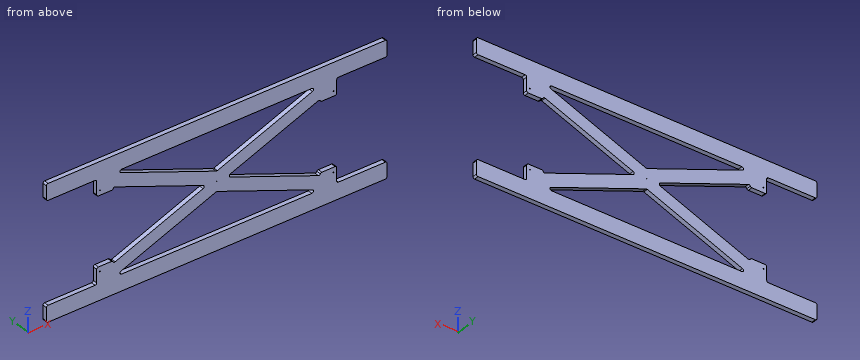
```python
from build123d import *

# Parameters (mm, degrees)
SKETCH1_W                    = 1333.5
SKETCH1_H                    = 520.7
BOSS_EXTRUDE1_DEPTH          = 17.78
FILLET1_R                    = 6.35
F_1_8_0_125_DIAMETER_HOLE1_D = 3.175
SKETCH5_W                    = 152.4
SKETCH5_H                    = 393.7
CUT_EXTRUDE1_DEPTH           = 18.78
FILLET2_R                    = 6.35
SKETCH6_W                    = 50.8
SKETCH6_H                    = 393.7
SKETCH6_W_2                  = 63.5
SKETCH6_H_2                  = 266.7
CUT_EXTRUDE2_DEPTH           = 18.78
FILLET3_R                    = 6.35


with BuildPart() as part:
    # Sketch1 → Boss-Extrude1 (new body)
    with BuildSketch(Plane(origin=(0, 0, 0), x_dir=(1, 0, 0), z_dir=(0, 1, 0))):
        Rectangle(SKETCH1_W, SKETCH1_H)
    extrude(amount=BOSS_EXTRUDE1_DEPTH)

    # Fillet1
    fillet1_edges = [part.edges().sort_by_distance(p)[0] for p in [
        (666.75, 8.89, 260.35),
        (-666.75, 8.89, 260.35),
        (-666.75, 8.89, -260.35),
        (666.75, 8.89, -260.35),
    ]]
    fillet(fillet1_edges, radius=FILLET1_R)

    # 1/8 (0.125) Diameter Hole1 (through all)
    with Locations(Plane(origin=(0, 17.78, 0), x_dir=(1, 0, 0), z_dir=(0, 1, 0))):
        with Locations((0, 0), (457.2, 152.4), (-457.2, -152.4), (-457.2, 152.4), (457.2, -152.4)):
            Hole(F_1_8_0_125_DIAMETER_HOLE1_D / 2)

    # Sketch5 → Cut-Extrude1 (cut, through all)
    with BuildSketch(Plane(origin=(0, 17.78, 0), x_dir=(1, 0, 0), z_dir=(0, 1, 0))):
        Polygon((-406.4, 196.85), (406.4, 196.85), (0, 38.1), align=None)
        Polygon((0, -38.1), (-406.4, -196.85), (406.4, -196.85), align=None)
        Polygon((406.4, 143.8671875), (406.4, -143.8671875), (38.1, 0), align=None)
        Polygon((-406.4, 143.8671875), (-38.1, 0), (-406.4, -143.8671875), align=None)
        with Locations((546.1, 0)):
            Rectangle(SKETCH5_W, SKETCH5_H)
        with Locations((-546.1, 0)):
            Rectangle(SKETCH5_W, SKETCH5_H)
    extrude(amount=-CUT_EXTRUDE1_DEPTH, mode=Mode.SUBTRACT)

    # Fillet2
    fillet2_edges = [part.edges().sort_by_distance(p)[0] for p in [
        (-406.4, 8.89, 143.8671875),
        (-406.4, 8.89, -143.8671875),
        (-38.1, 8.89, 0),
        (622.3, 8.89, -196.85),
        (622.3, 8.89, 196.85),
        (469.9, 8.89, 196.85),
        (469.9, 8.89, -196.85),
        (0, 8.89, 38.1),
        (406.4, 8.89, 196.85),
        (-406.4, 8.89, 196.85),
        (38.1, 8.89, 0),
        (406.4, 8.89, -143.8671875),
        (406.4, 8.89, 143.8671875),
        (406.4, 8.89, -196.85),
        (0, 8.89, -38.1),
        (-406.4, 8.89, -196.85),
        (-469.9, 8.89, -196.85),
        (-469.9, 8.89, 196.85),
        (-622.3, 8.89, 196.85),
        (-622.3, 8.89, -196.85),
    ]]
    fillet(fillet2_edges, radius=FILLET2_R)

    # Sketch6 → Cut-Extrude2 (cut, through all)
    with BuildSketch(Plane(origin=(0, 17.78, 0), x_dir=(1, 0, 0), z_dir=(0, 1, 0))):
        with Locations((641.35, 0)):
            Rectangle(SKETCH6_W, SKETCH6_H)
        with Locations((-641.35, 0)):
            Rectangle(SKETCH6_W, SKETCH6_H)
        with Locations((-438.15, 0)):
            Rectangle(SKETCH6_W_2, SKETCH6_H_2)
        with Locations((438.15, 0)):
            Rectangle(SKETCH6_W_2, SKETCH6_H_2)
    extrude(amount=-CUT_EXTRUDE2_DEPTH, mode=Mode.SUBTRACT)

    # Fillet3
    fillet3_edges = [part.edges().sort_by_distance(p)[0] for p in [
        (-666.75, 8.89, 196.85),
        (-666.75, 8.89, -196.85),
        (666.75, 8.89, -196.85),
        (666.75, 8.89, 196.85),
        (-406.4, 8.89, 133.35),
        (-406.4, 8.89, -133.35),
        (-469.9, 8.89, 133.35),
        (-469.9, 8.89, -133.35),
        (469.9, 8.89, -133.35),
        (406.4, 8.89, -133.35),
        (469.9, 8.89, 133.35),
        (406.4, 8.89, 133.35),
    ]]
    fillet(fillet3_edges, radius=FILLET3_R)


solid = part.part
```
Input: part model. Units: mm. Frame: model coordinates. Coordinates: 2 decimals unless noted, no trailing zeros. Loops run counter-clockwise (first coordinate to the right, second up) from the corner with the lowest first, then second, coordinate; pieces in that order, holes last. Notation, with made-up numbers: (29, 9.5) -> (46, 9.5) arc R33 cw to (46, 42.5) -> close; hole circle Ø1 at (46, 30.25). An arc over 180 degrees is marked (long way). Use a Markdown table: item, result.
1) Cut plane C-C (y = 14.5). Give the number of separate pieces and of enclosed holes in the cut face, then the cut area to 3 significant figures.
Results found:
| item | result |
|---|---|
| separate pieces | 1 |
| enclosed holes | 7 |
| area | 271,000 mm2 |
2) Cut plane B-B (x = -297). Return the cut outline in (y, z), then the cut area to 3 significant figures.
Results found:
| item | result |
|---|---|
| outline | (0, -260.35) -> (17.78, -260.35) -> (17.78, -196.85) -> (0, -196.85) -> close; (0, -154.12) -> (17.78, -154.12) -> (17.78, -101.13) -> (0, -101.13) -> close; (0, 101.13) -> (17.78, 101.13) -> (17.78, 154.12) -> (0, 154.12) -> close; (0, 196.85) -> (17.78, 196.85) -> (17.78, 260.35) -> (0, 260.35) -> close |
| area | 4,140 mm2 |
3) Cut plane D-D (z = 172.5). Return the cut outline in (x, y).
Results found:
| item | result |
|---|---|
| outline | (-469.9, 0) -> (-344.06, 0) -> (-344.06, 17.78) -> (-469.9, 17.78) -> close; (344.06, 0) -> (469.9, 0) -> (469.9, 17.78) -> (344.06, 17.78) -> close |
4) Material intervals for line 1 along Z through (x, y) = (-457.2, 5.75); line 2 along Z through (x, y) = (130, 8); line 3 along Z through (x, y) = (9, 5.5), sorted ascending. Write a range as from..to.
Results found:
| item | result |
|---|---|
| line 1 | z = -260.35..-153.99, -150.81..-133.35, 133.35..150.81, 153.99..260.35 |
| line 2 | z = -260.35..-196.85, -88.88..-35.9, 35.9..88.88, 196.85..260.35 |
| line 3 | z = -260.35..-196.85, -41.62..41.62, 196.85..260.35 |
5) Contact query for flat-ended pins moving along their axis: pin 1 (2.5 mm diameter, centred on x = 457.2, z = -152.4, fed in from -Y); pin 2 (3 mm diameter, centred on y = 8.5, z = 193, fed in from -X); pin 3 (9 mm diameter, centred on y = 9, z = -162.5, fed in from +X). Output: stop coordinate, or through.
Results found:
| item | result |
|---|---|
| pin 1 | passes through |
| pin 2 | stops at x = -471.32 |
| pin 3 | stops at x = 469.9 |
6) Cut plane A-A (z = -108). Return the cut outline in (x, y).
Results found:
| item | result |
|---|---|
| outline | (-314.58, 0) -> (-178.94, 0) -> (-178.94, 17.78) -> (-314.58, 17.78) -> close; (178.94, 0) -> (314.58, 0) -> (314.58, 17.78) -> (178.94, 17.78) -> close |
